from build123d import *

# Parameters (mm, degrees)
F1_ANGLE = 30


with BuildPart() as f1:
    # F0 (on Front) → F1 (revolve, symmetric)
    with BuildSketch(Plane.XZ) as f1_sk:
        Polygon((-38.094878, 28.946124), (-38.094878, 20.847209), (38.094878, 20.847209), (38.094878, 28.946124), (17.997593, 28.946124), (17.997593, 50.543226), (27.596295, 50.543226), (27.596295, 60.591869), (-25.946513, 60.591869), (-25.946513, 52.942902), (-7.049054, 52.942902), (-7.049054, 28.946124), align=None)
    revolve(axis=Axis((1.79977, 0, 0), (1, 0, 0)), revolution_arc=F1_ANGLE / 2)
    revolve(f1_sk.sketch, axis=Axis((1.79977, 0, 0), (-1, 0, 0)), revolution_arc=F1_ANGLE / 2)


solid = f1.part
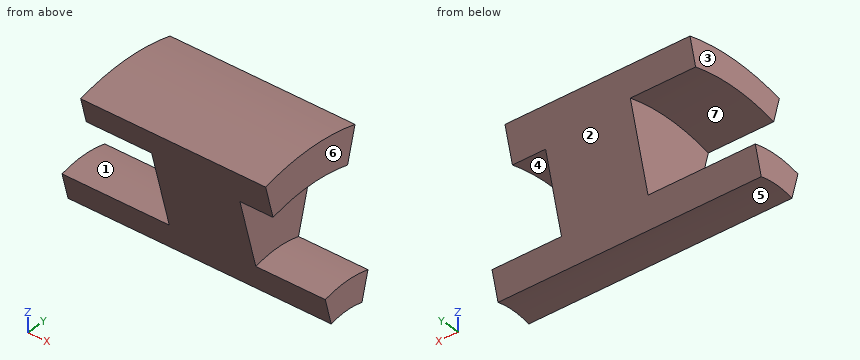
Source: CAD feature listing. Evaluate the final solid. Frame: model axes, mm. Face numbers are marked on the shaded views. A direction names the side the tool comes from. Coordinates: 2 decimals unless noted, no trailing zeros. Order: outer loops, then holes, each group sorted by start corner. A loop starts at its lowest first (then second) coordinate and runs counter-clockwise, first axis right, second up. Notation, with made-up numbers: M 29,25 L 79,25 A12 ccw 79,34 Z; hole C -14.5,84.25 d8. An arc over 180 degrees is marked long. Write each question's results on one line, items separated by ' | '. Start each with the question number.
1. Section A-A, the plane x = -16. Return the cut outline in (y, z), then the cut area to 3 significant figures.
2. Draft query along Z for the marked faces 5, 6 and 7. Return one class per face: +Z half, -Z half, draft (parallel to the pull), parting line (faces both ways), or undercut.
3. Pin query (flat end, axial travel): pin 1 (4 mm diameter, centred on x = 17.5, z = 30.5, fed in from +Y); pin 2 (10 mm diameter, centred on x = -19.5, z = 32.5, fed in from +Y); pin 3 (1.5 mm diameter, centred on y = 4.5, z = 55, fed in from +X); pin 4 (18 mm diameter, centred on y = 1, z = 34.5, fed in from +X). Return the tip coordinate at first contact, or that it passes through.
4. Material intervals for L1, parallel to X at y = -6.5, z = 42; L2, parallel to Z at x = 31, y = 0.5; L3, parallel to X at y = -3, z = 57, sorted ascending.
5. Section B-B, the plane y = 0. Return the cut outline in (x, z), then the cut area to 3 significant figures.
6. Section D-D, the plane y = -3.5. Return the cut outline in (x, z).
7. Reachability of the marked faces 1, 2, 3 and 4 from +Z, -Z, +X, -X, +Y, -Y: full face, straight path, thin tool, end or side. Return the list, or none.
8. Section C-C, the plane x = 9. Return the cut outline in (y, z), then the cut area to 3 significant figures.
Solution:
1) outline: M -15.68,58.53 L -13.7,51.14 A52.94 cw 13.7,51.14 L 15.68,58.53 A60.59 ccw Z; M -7.49,27.96 L -5.4,20.14 A20.85 cw 5.4,20.14 L 7.49,27.96 A28.95 ccw Z | area: 333 mm²
2) face 5: -Z half | face 6: draft | face 7: undercut
3) pin 1: y = 8.71 | pin 2: y = 7.49 | pin 3: x = 27.6 | pin 4: x = 38.09
4) L1: -7.05 to 18 | L2: 20.84 to 28.94 | L3: -25.95 to 27.6
5) outline: M -38.09,20.85 L 38.09,20.85 L 38.09,28.95 L 18,28.95 L 18,50.54 L 27.6,50.54 L 27.6,60.59 L -25.95,60.59 L -25.95,52.94 L -7.05,52.94 L -7.05,28.95 L -38.09,28.95 Z | area: 1,650 mm²
6) outline: M -38.09,20.55 L 38.09,20.55 L 38.09,28.73 L 18,28.73 L 18,50.42 L 27.6,50.42 L 27.6,60.49 L -25.95,60.49 L -25.95,52.83 L -7.05,52.83 L -7.05,28.73 L -38.09,28.73 Z
7) face 1: -X | face 2: -Z, +X, -X, +Y | face 3: +Z, -X, +Y, -Y | face 4: +X
8) outline: M -15.68,58.53 L -5.4,20.14 A20.85 cw 5.4,20.14 L 15.68,58.53 A60.59 ccw Z | area: 847 mm²
